Work out the finished part from the listing and answer in its coordinate system (mm). A direction names the side the tool comes from. Coordinates: 2 decimals unless noted, no trailing zeros. Order: outer loops, then holes, each group sorted by start corner. A loop starts at its lowest first (then second) coordinate and runs counter-clockwise, first axis right, second up. Notation, with made-up numbers: M 1.25,-28.5 L 47.25,-28.5 A32 ccw 47.25,5.5 Z; hole C 56.5,79.25 d1. An arc over 180 degrees is marked long. Use a Markdown table: item, result.
from build123d import *

# Parameters (mm, degrees)
F1_DEPTH = 19
F2_W     = 6.5
F2_H     = 68
F3_DEPTH = 20
F4_W     = 6.5
F4_H     = 68
F5_DEPTH = 20


with BuildPart() as f1:
    # F0 (on Front) → F1 (new body)
    with BuildSketch(Plane.XZ):
        Polygon((-65.72042, 69.094742), (-85.72042, 69.094742), (-85.72042, 1.094742), (-65.72042, 1.094742), (-65.72042, -10.905258), (232.27958, -10.905258), (232.27958, 1.094742), (252.27958, 1.094742), (252.27958, 69.094742), (232.27958, 69.094742), (232.27958, 81.094742), (-65.72042, 81.094742), align=None)
    extrude(amount=F1_DEPTH)

    # F2 (on face) → F3 (cut)
    with BuildSketch(Plane.YZ.offset(252.27958)):
        with Locations((-15.75, 35.094742)):
            Rectangle(F2_W, F2_H)
        with Locations((-3.25, 35.094742)):
            Rectangle(F2_W, F2_H)
    extrude(amount=-F3_DEPTH, mode=Mode.SUBTRACT)

    # F4 (on face) → F5 (cut)
    with BuildSketch(Plane(origin=(-85.72042, 0, 0), x_dir=(0, -1, 0), z_dir=(-1, 0, 0))):
        with Locations((3.25, 35.094742)):
            Rectangle(F4_W, F4_H)
        with Locations((15.75, 35.094742)):
            Rectangle(F4_W, F4_H)
    extrude(amount=-F5_DEPTH, mode=Mode.SUBTRACT)


solid = f1.part
1. For faces 1 (the face through (-76, -9, 1.095)), 2 (the face through (242, -12.5, 35)), 3 (the face through (242, -9, 1.095)), 4 (the face through (-76, -12.5, 35)), 5 (the face through (-76, -6.5, 35)), determine the directions among +Z, -Z, +X, -X, +Y, -Y from which every point of the face is accessible in a straight line to the end or side of a thin tool.
Answers below:
| item | result |
|---|---|
| face 1 | -Z, -X, +Y, -Y |
| face 2 | +Z, -Z, +X, -Y |
| face 3 | -Z, +X, +Y, -Y |
| face 4 | +Z, -Z, -X, -Y |
| face 5 | +Z, -Z, -X, +Y |
2. Flat-ended cylindrical pins translate along their axes: P1, Ø10, axis at x = 245.5, z = 35, coming from the +Y side; P2, Ø5, axis at x = -78, y = -9, coming from the -Z side; P3, Ø3, axis at x = -79.5, y = -8.5, coming from the +Z side. Find the tip coordinate at first contact, or state that the pin passes through.
Answers below:
| item | result |
|---|---|
| P1 | y = -6.5 |
| P2 | z = 1.09 |
| P3 | z = 69.09 |
3. Find the intervals of material crossed by probe 1 along X at (y, z) = (-14, 28.5); probe 2 along Y at (x, z) = (233.5, 7.5), in increasing order.
Answers below:
| item | result |
|---|---|
| probe 1 | -65.72 to 232.28 |
| probe 2 | -12.5 to -6.5 |
4. Section A-A on z = 18 is taken. Determine the outline of the cut face in (x, y).
Answers below:
| item | result |
|---|---|
| outline | M -85.72,-12.5 L -65.72,-12.5 L -65.72,-19 L 232.28,-19 L 232.28,-12.5 L 252.28,-12.5 L 252.28,-6.5 L 232.28,-6.5 L 232.28,0 L -65.72,0 L -65.72,-6.5 L -85.72,-6.5 Z |
